from build123d import *

# Parameters (mm, degrees)
SALIENTE_EXTRUIR1_DEPTH = 40
CROQUIS2_R              = 2.5
CORTAR_EXTRUIR1_DEPTH   = 22.5
CORTAR_EXTRUIR5_DEPTH   = 14
CROQUIS6_R              = 4
CROQUIS6_R_2            = 2.5
SALIENTE_EXTRUIR2_DEPTH = 1


with BuildPart() as part:
    # Croquis1 → Saliente-Extruir1 (new body)
    with BuildSketch(Plane.XY):
        with BuildLine():
            ThreePointArc((-13.23096405, 11.648445498), (-13.584517441, 11.501998889), (-13.73096405, 11.148445498))
            Line((-13.73096405, 11.148445498), (-13.73096405, 2.035658412))
            ThreePointArc((-13.73096405, 2.035658412), (-13.626281451, 1.729514406), (-13.356067441, 1.551562201))
            Line((-13.356067441, 1.551562201), (-12.169475815, 1.244915231))
            ThreePointArc((-12.169475815, 1.244915231), (-11.899261805, 1.066963026), (-11.794579206, 0.76081902))
            Line((-11.794579206, 0.76081902), (-11.794579206, 0.442917518))
            ThreePointArc((-11.794579206, 0.442917518), (-11.736179814, 0.265071669), (-11.583718232, 0.156466416))
            ThreePointArc((-11.583718232, 0.156466416), (-7.701884055, -0.773383829), (-3.73096405, -1.17965021))
            ThreePointArc((-3.73096405, -1.17965021), (0.239955955, -0.773383829), (4.121790132, 0.156466416))
            ThreePointArc((4.121790132, 0.156466416), (4.274251714, 0.265071669), (4.332651106, 0.442917518))
            Line((4.332651106, 0.442917518), (4.332651106, 0.76081902))
            ThreePointArc((4.332651106, 0.76081902), (4.437333704, 1.066963026), (4.707547715, 1.244915231))
            Line((4.707547715, 1.244915231), (5.894139341, 1.551562201))
            ThreePointArc((5.894139341, 1.551562201), (6.164353351, 1.729514406), (6.26903595, 2.035658412))
            Line((6.26903595, 2.035658412), (6.26903595, 11.148445498))
            ThreePointArc((6.26903595, 11.148445498), (6.12258934, 11.501998889), (5.76903595, 11.648445498))
            Line((5.76903595, 11.648445498), (3.76903595, 11.648445498))
            ThreePointArc((3.76903595, 11.648445498), (3.415482559, 11.501998889), (3.26903595, 11.148445498))
            Line((3.26903595, 11.148445498), (3.26903595, 10.648445498))
            ThreePointArc((3.26903595, 10.648445498), (-0.206558338, 10.028093004), (-3.73096405, 9.82034979))
            ThreePointArc((-3.73096405, 9.82034979), (-7.255369763, 10.028093004), (-10.73096405, 10.648445498))
            Line((-10.73096405, 10.648445498), (-10.73096405, 11.148445498))
            ThreePointArc((-10.73096405, 11.148445498), (-10.87741066, 11.501998889), (-11.23096405, 11.648445498))
            Line((-11.23096405, 11.648445498), (-13.23096405, 11.648445498))
        make_face()
    extrude(amount=SALIENTE_EXTRUIR1_DEPTH)

    # Croquis2 → Cortar-Extruir1 (cut, symmetric)
    with BuildSketch(Plane(origin=(0, 0, 0), x_dir=(1, 0, 0), z_dir=(0, 1, 0))):
        with Locations(Location((-3.73096405, -30, 0), (0, 0, 90))):
            Circle(CROQUIS2_R)
        with BuildLine():
            Line((-13.73096405, -30), (-13.73096405, -43.289358514))
            Line((-13.73096405, -43.289358514), (6.26903595, -43.289358514))
            Line((6.26903595, -43.289358514), (6.26903595, -30))
            ThreePointArc((6.26903595, -30), (-3.73096405, -40), (-13.73096405, -30))
        make_face()
    extrude(amount=CORTAR_EXTRUIR1_DEPTH, both=True, mode=Mode.SUBTRACT)

    # Croquis5 → Cortar-Extruir5 (cut)
    with BuildSketch(Plane(origin=(0, 1.648445498, 0), x_dir=(1, 0, 0), z_dir=(0, 1, 0))):
        with BuildLine():
            Line((-13.73096405, 0), (-13.73096405, -40.777418578))
            Line((-13.73096405, -40.777418578), (6.26903595, -40.777418578))
            Line((6.26903595, -40.777418578), (6.26903595, 0))
            ThreePointArc((6.26903595, 0), (-3.73096405, -10), (-13.73096405, 0))
        make_face()
    extrude(amount=-CORTAR_EXTRUIR5_DEPTH, mode=Mode.SUBTRACT)

    # Croquis6 → Saliente-Extruir2 (add)
    with BuildSketch(Plane.XZ.offset(-1.648445498)):
        with Locations(Location((-3.73096405, 30, 0), (0, 0, 180))):
            Circle(CROQUIS6_R)
        with Locations(Location((-3.73096405, 30, 0), (0, 0, 270))):
            Circle(CROQUIS6_R_2, mode=Mode.SUBTRACT)
    extrude(amount=SALIENTE_EXTRUIR2_DEPTH)


solid = part.part
For this review, take the finished solid that the model builds, in its own axes (mm). A direction names the side the tool comes from. Round coordinates to 2 decimals unless told otherwise and drop trailing zeros. Write each loop counter-clockwise with the first axis right and the second up, starting at its lowest first coordinate (ties: lowest second). Pieces come first, ordered by that corner, then holes. Notation, with made-up numbers: (71.25, 74) - (107.25, 74) arc R24 ccw to (107.25, 106) - close; hole circle Ø11 at (-5.75, -38). An arc over 180 degrees is marked (long way). Write item = value, one per line. Start each with the question number.
1. Consider section C-C on z = 34.5. State the section outline as (x, y) points, plus the area to 3 significant figures.
2. Wall thickness on L1, parallel to X at y = 0.9, z = 30; L2, parallel to X at y = 6.75, z = 30; L3, parallel to Y at x = 4.5, z = 11: over which ranges is each line inside the solid? List them lowest first.
3. For faces 1 (the face through (-12.77, 1.4, 2.05)), 2 (the face through (-4, 0.648, 33)), 3 (the face through (-3.54, 0.57, 10)), list the 3-axis set-ups (+Z, -Z, +X, -X, +Y, -Y) from which the entire face can be reached by the end or side of a thin tool; tool diameter is ignored.
4. Consider section B-B on y = 8.5. State the section outline as (x, z) points.
5. For pin 1 Ø2 at (x, z) = (-2.5, 23.5) entering from -Y; pin 2 Ø6.5 at (x, z) = (-3.73, 30) entering from +Y; pin 3 Ø6.5 at (x, z) = (-3.73, 30) entering from -Y, all flat-tipped, find the tip position at first contact; note any pin that passes through.
6. Consider section A-A on z = 14.5. State the section outline as (x, y) points.
Evaluation:
q1.outline = (-12.66, 1.65) - (5.2, 1.65) - (5.2, 11.65) - (3.77, 11.65) arc R0.5 ccw to (3.27, 11.15) - (3.27, 10.65) arc R30 cw to (-10.73, 10.65) - (-10.73, 11.15) arc R0.5 ccw to (-11.23, 11.65) - (-12.66, 11.65) - close
q1.area = 157 mm2
q2.L1 = -7.73 to -6.23, -1.23 to 0.27
q2.L2 = -13.73 to -6.23, -1.23 to 6.27
q2.L3 = 1.65 to 11.65
q3.face_1 = +Z, -Z, -X, -Y
q3.face_2 = +Z, +X, -X, -Y
q3.face_3 = -Y
q4.outline = (-13.73, 0) - (6.27, 0) - (6.27, 30) arc R10 ccw to (-13.73, 30) - close; hole circle Ø5 at (-3.73, 30)
q5.pin_1 = 1.65
q5.pin_2 = 10
q5.pin_3 = 0.65
q6.outline = (-13.73, 2.04) arc R0.5 ccw to (-13.55, 1.65) - (6.09, 1.65) arc R0.5 ccw to (6.27, 2.04) - (6.27, 11.15) arc R0.5 ccw to (5.77, 11.65) - (3.77, 11.65) arc R0.5 ccw to (3.27, 11.15) - (3.27, 10.65) arc R30 cw to (-10.73, 10.65) - (-10.73, 11.15) arc R0.5 ccw to (-11.23, 11.65) - (-13.23, 11.65) arc R0.5 ccw to (-13.73, 11.15) - close
